The drawing under review shows one solid part. Ordinate dimensions are in mm from its lowest x, y, z. Round coordinates to 2 decimals unless told otherwise and drop trailing zeros. Order: outer loops, then holes, each group sorted by start corner. A loop starts at its lowest first (then second) coordinate and runs counter-clockwise, first axis right, second up. Notation, with made-up numbers: M -1,-11.75 L 41,-11.75 A14 ccw 41,2.25 Z; hole C -11.75,46.5 d4. An arc over 180 degrees is marked long. Write item = value, one per line. Start each with the question number.
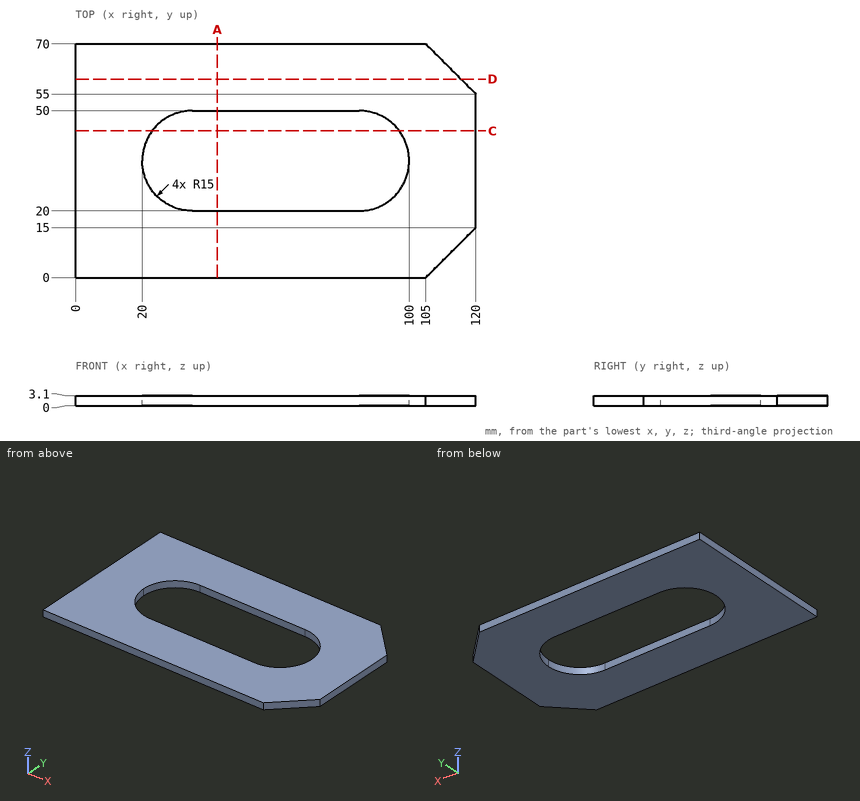
(1) Consider section D-D, the plane y = 59.5. Write out the cut boundary in (x, z).
(2) For line 1 along Y through (x, z) = (43.5, 0.25); line 2 along X through (y, z) = (46, 1.4); line 3 along Y through (x, z) = (89.5, 2.75), list the stretches that pass through material, from the lowest coordinate up. Write a range as [from, to].
(3) Consider section C-C, the plane y = 44. Write out the cut boundary in (x, z), then the cut area to 3 significant figures.
(4) Consider section A-A, the plane x = 42.5. Write out the cut boundary in (y, z), then the cut area to 3 significant figures.
Completed:
q1.outline = M 0,0 L 115.5,0 L 115.5,3.1 L 0,3.1 Z
q2.line_1 = [0, 20], [50, 70]
q2.line_2 = [0, 24.8], [95.2, 120]
q2.line_3 = [0, 20.69], [49.31, 70]
q3.outline = M 0,0 L 23,0 L 23,3.1 L 0,3.1 Z; M 97,0 L 120,0 L 120,3.1 L 97,3.1 Z
q3.area = 143 mm2
q4.outline = M 0,0 L 20,0 L 20,3.1 L 0,3.1 Z; M 50,0 L 70,0 L 70,3.1 L 50,3.1 Z
q4.area = 124 mm2
